Design review of the part built by this model. Coordinates are the model's own, in mm. A direction names the side the tool comes from. Coordinates: 2 decimals unless noted, no trailing zeros. Order: outer loops, then holes, each group sorted by start corner. A loop starts at its lowest first (then second) coordinate and runs counter-clockwise, first axis right, second up. Notation, with made-up numbers: (17, -22.5) -> (21, -22.5) arc R25 cw to (21, 5.5) -> close; hole circle Ø2 at (17.5, 69.5). An arc over 180 degrees is marked (long way). Use a Markdown table: item, result. Add a question column.
Q1. Add section A-A (y = 2). State the section outline as (x, z) points, then the cut area to 3 significant figures.
Q2. The part is to be moulded in two halves that separate along X. For faces 4 (the face through (-32, 0, -1)), 5 (the face through (0, 7, -1)), 6 (the face through (-50, 4, -1)), 7 (the face through (-15, 2, -1)), say which applies: pulls with the +X half, pulls with the -X half, needs draft (parallel to the pull), parting line crosses it, or undercut.
Q3. Add section C-C (x = -7). State the section outline as (y, z) points.
Q4. Machinability: for faces 1 (the face through (15, 3, -1)), 2 (the face through (1, 8, 55)), 3 (the face through (18, 5, -1)), which of the approach directions +Z, -Z, +X, -X, +Y, -Y give a long, thin tool a straight path to every point of the face, cutting with its end or side? Answer none if there is none.
Q5. Add section D-D (x = -30.5). State the section outline as (y, z) points.
Q6. Add section B-B (z = -37.5). State the section outline as (x, y) points, then the cut area to 3 significant figures.
Q7. Wall thickness on probe 1 along X at (y, z) = (4.75, -29); probe 2 along Y at (x, z) = (-17, -15); probe 3 along Z at (x, y) = (5.5, 9.5): over which ranges is each line inside the solid? List them lowest first.
Q8. Insertion check: pin 1 (1 mm diameter, centred on x = -1.5, y = 10, fed in from +Z); pin 2 (1 mm diameter, centred on y = 10.5, z = 3.5, fed in from -X); pin 3 (10 mm diameter, centred on x = 34.5, z = -42, fed in from +Y). Each pin has a flat end and moves straight along its axis. Give the tip position at first contact, or say it passes through.
from build123d import *

# Parameters (mm, degrees)
SKETCH2_W          = 100
SKETCH2_H          = 9
EXTRUDE1_DEPTH     = 55
CUT_EXTRUDE1_DEPTH = 111
SKETCH7_W          = 40
SKETCH7_H          = 20
EXTRUDE2_DEPTH     = 2


with BuildPart() as part:
    # Sketch2 → Extrude1 (new body, symmetric)
    with BuildSketch(Plane(origin=(0, 0, 0), x_dir=(-1, 0, 0), z_dir=(0, 0, -1))):
        with Locations((0, 4.5)):
            Rectangle(SKETCH2_W, SKETCH2_H)
    extrude(amount=EXTRUDE1_DEPTH, both=True)

    # Sketch5 → Cut-Extrude1 (cut, through all)
    with BuildSketch(Plane(origin=(0, 0, -55), x_dir=(-1, 0, 0), z_dir=(0, 0, -1))):
        Polygon((20, 5), (20, 7), (-20, 7), (-20, 5), (-15, 5), (-15, 0), (15, 0), (15, 5), align=None)
    extrude(amount=-CUT_EXTRUDE1_DEPTH, mode=Mode.SUBTRACT)

    # Sketch7 → Extrude2 (add)
    with BuildSketch(Plane(origin=(0, 9, 0), x_dir=(1, 0, 0), z_dir=(0, 1, 0))):
        Rectangle(SKETCH7_W, SKETCH7_H)
    extrude(amount=EXTRUDE2_DEPTH)


solid = part.part
Established:
| question | item | result |
|---|---|---|
| 1 | outline | (-50, -55) -> (-15, -55) -> (-15, 55) -> (-50, 55) -> close; (15, -55) -> (50, -55) -> (50, 55) -> (15, 55) -> close |
| 1 | area | 7,700 mm^2 |
| 2 | face 4 | needs draft |
| 2 | face 5 | undercut |
| 2 | face 6 | pulls with the -X half |
| 2 | face 7 | undercut |
| 3 | outline | (7, -55) -> (9, -55) -> (9, -10) -> (11, -10) -> (11, 10) -> (9, 10) -> (9, 55) -> (7, 55) -> close |
| 4 | face 1 | +Z, -Z, -Y |
| 4 | face 2 | +Z, +X, -X, +Y, -Y |
| 4 | face 3 | +Z, -Z |
| 5 | outline | (0, -55) -> (9, -55) -> (9, 55) -> (0, 55) -> close |
| 6 | outline | (-50, 0) -> (-15, 0) -> (-15, 5) -> (-20, 5) -> (-20, 7) -> (20, 7) -> (20, 5) -> (15, 5) -> (15, 0) -> (50, 0) -> (50, 9) -> (-50, 9) -> close |
| 6 | area | 670 mm^2 |
| 7 | probe 1 | -50 to -15, 15 to 50 |
| 7 | probe 2 | 0 to 5, 7 to 9 |
| 7 | probe 3 | -10 to 10 |
| 8 | pin 1 | z = 10 |
| 8 | pin 2 | x = -20 |
| 8 | pin 3 | y = 9 |
